Autodesk Inventor part; units mm, degrees
ref_plane "Work Plane1" through (125.8734, -33.1867, 0) normal (0.5, 0.866, 0) x (0.866, -0.5, 0)
ref_plane "YZ Plane" through (0, 0, 0) normal (1, 0, 0) x (0, 1, 0)
ref_plane "XZ Plane" through (0, 0, 0) normal (0, 1, 0) x (-1, 0, 0)
sketch "Sketch1" plane through (0, 0, 0) normal (0, 0, 1) x (1, 0, 0)
  line L0 (0, 0) -> (58, 0)
  line L1 (58, 0) -> (58, 12)
  line L2 (58, 12) -> (0, 12)
  line L3 (0, 12) -> (0, 0)
  line L4 (58, 12) -> (36.0591, 24.6676) construction
  line L5 (58, 12) -> (129.0141, -29)
  line L6 (58, 12) -> (140, 12) construction
  line L7 (58, 0) -> (123.8179, -38)
  line L8 (58, 0) -> (134, 0) construction
  line L9 (123.8179, -38) -> (128.4714, -28.6867)
  dimension "d0" = 58
  dimension "d1" = 12
  dimension "d2" = 30
  dimension "d3" = 82
  dimension "d4" = 30
  dimension "d5" = 30
  dimension "d6" = 93.45
  dimension "d7" = 127.746
  dimension "d8" = 106.5151
extrude "Extrusion1" add sketch "Sketch1" against normal blind 52
ref_plane "Work Plane1" through (125.8734, -33.1867, 0) normal (0.5, 0.866, 0) x (0.866, -0.5, 0)
sketch "Sketch3" plane through (125.8734, -33.1867, 0) normal (0.5, 0.866, 0) x (0.866, -0.5, 0)
  line L0 (0, 0) -> (0, 52) construction
  circle A0 centre (0, 26) radius 26
  circle A1 centre (0, 26) radius 13
  point P0 (-125.6029, 0)
  dimension "d12" = 26
extrude "Extrusion2" add sketch "Sketch3" along normal mid plane 16
extrude "Extrusion3" cut sketch "Sketch3" along normal through all both and the other way through all contours A1
sketch "Sketch4" plane through (0, 12, 0) normal (0, 1, 0) x (1, 0, 0)
  line L0 (0, 0) -> (0, 52)
  line L1 (0, 26) -> (0, 39)
  line L2 (0, 39) -> (32, 39)
  line L3 (32, 39) -> (32, 13)
  line L4 (32, 13) -> (0, 13)
  line L5 (0, 13) -> (0, 39)
  dimension "d17" = 13
  dimension "d18" = 32
  dimension "d19" = 26
extrude "Extrusion4" cut sketch "Sketch4" against normal through all
fillet "Fillet1" radius 12 2 edges at (0, 6, 0) (0, 6, -52)
properties part number "LE-1.4"
Can you work these out from the model? Positions are in its coordinate system, mm. A direction names the side the tool comes from. Coordinates: 2 decimals unless noted, no trailing zeros. Loops run counter-clockwise (first coordinate to the right, second up) from the corner with the lowest first, then second, coordinate; pieces in that order, holes last. Notation, with made-up numbers: (9.25, 1.25) -> (43.25, 1.25) arc R21 cw to (43.25, 30.25) -> close; hole circle Ø8 at (-29.75, 81.25). An arc over 180 degrees is marked (long way). Answer as a JSON object with one key per item and string values.
1) For faces 4 (the face through (32, 6, -26)), 5 (the face through (36, 12, -26)), 6 (the face through (35, 0, -26)), which set-ups out of +Z, -Z, +X, -X, +Y, -Y let a thin tool reach every point of the face, with its end or its side?
Results:
{"face 4": "-X, +Y, -Y", "face 5": "+Z, -Z, +X, -X, +Y", "face 6": "+Z, -Z, -X, -Y"}
2) Imagine slicing it at A-A (x = 29). Please give me the cut outline in (y, z), then the cut area to 3 significant figures.
Results:
{"outline": "(0, -52) -> (12, -52) -> (12, -39) -> (0, -39) -> close; (0, -13) -> (12, -13) -> (12, 0) -> (0, 0) -> close", "area": "312 mm^2"}
3) Thinking about a two-plate mould opening in Y: for faces 1 (the face through (147.294, -45.683, -18.19)), 2 (the face through (70, -5, -52)), 3 (the face through (84.912, -3.538, -25.636)), which applies, pulls with the +Y half, pulls with the -Y half, needs draft (parallel to the pull), parting line crosses it, or undercut?
Results:
{"face 1": "undercut", "face 2": "needs draft", "face 3": "pulls with the +Y half"}
4) Imagine slicing it at B-B (z = -37). Please give me the cut outline in (x, y), then the cut area to 3 significant figures.
Results:
{"outline": "(32, 0) -> (58, 0) -> (102.87, -25.91) -> (101.47, -28.34) -> (115.87, -36.65) -> (123.87, -22.79) -> (109.47, -14.48) -> (108.07, -16.91) -> (58, 12) -> (32, 12) -> close; (127.87, -43.58) -> (142.28, -51.89) -> (150.28, -38.04) -> (135.87, -29.72) -> close", "area": "1,410 mm^2"}
5) Imagine slicing it at C-C (y = 3.5). Please give me the cut outline in (x, z).
Results:
{"outline": "(0, -40) arc R12 ccw to (12, -52) -> (72.72, -52) -> (72.72, 0) -> (12, 0) arc R12 ccw to (0, -12) -> (0, -13) -> (32, -13) -> (32, -39) -> (0, -39) -> close"}
6) If I drill on line 1 (Y direction, x = 39.5, z = -41); line 2 (Y direction, x = 146.5, z = -32.5); line 3 (X direction, y = -2, z = -35), over which ranges is the centre line in solid material (lowest first)?
Results:
{"line 1": "y = 0 to 12", "line 2": "y = -47.81 to -35.86", "line 3": "x = 61.46 to 82.25"}
7) Imagine slicing it at D-D (z = -6.5). Please give me the cut outline in (x, y).
Results:
{"outline": "(1.33, 0) -> (58, 0) -> (108.38, -29.09) -> (106.98, -31.52) -> (136.77, -48.71) -> (144.77, -34.86) -> (114.98, -17.66) -> (113.58, -20.09) -> (58, 12) -> (1.33, 12) -> close"}
8) For P1, Ø12, axis at y = -15.5, z = -19.5, coming from the +X side; P2, Ø13, axis at y = 3.5, z = -30, coming from the -X side; P3, Ø4, axis at y = -28, z = -19, coming from the +X side; P4, Ø10, axis at x = 86.5, y = -25.5, coming from the +Z side, each with a flat end and sliding along its axis, tell me the tip position at first contact or that it passes through.
Results:
{"P1": "stops at x = 121.18", "P2": "stops at x = 32", "P3": "stops at x = 118.33", "P4": "passes through"}
